from build123d import *

# Parameters (mm, degrees)
BOSS_EXTRUDE2_DEPTH     = 177.8
SKETCH19_R              = 2.2479
CUT_EXTRUDE3_DEPTH      = 27.67
SKETCH21_W              = 3.048
SKETCH21_H              = 14.224
BOSS_EXTRUDE4_DEPTH     = 14.224
SKETCH22_R              = 2.2479
CUT_EXTRUDE4_DEPTH      = 24.622
CUT_EXTRUDE4_DEPTH_BACK = 4.048


with BuildPart() as part:
    # Sketch2 → Boss-Extrude2 (new body)
    with BuildSketch(Plane.XY):
        with BuildLine():
            Line((0, 0), (0, 22.86))
            Line((0, 22.86), (26.67, 22.86))
            Line((26.67, 22.86), (26.67, 0))
            Line((26.67, 0), (23.495, 0))
            Line((23.495, 0), (23.495, 18.542))
            ThreePointArc((23.495, 18.542), (22.974235857, 19.799235857), (21.717, 20.32))
            Line((21.717, 20.32), (4.953, 20.32))
            ThreePointArc((4.953, 20.32), (3.695764143, 19.799235857), (3.175, 18.542))
            Line((3.175, 18.542), (3.175, 0))
            Line((3.175, 0), (0, 0))
        make_face()
    extrude(amount=-BOSS_EXTRUDE2_DEPTH)

    # Sketch19 → Cut-Extrude3 (cut, through all)
    with BuildSketch(Plane(origin=(0, 0, 0), x_dir=(0, 0, -1), z_dir=(1, 0, 0))):
        with Locations((24.13, 9.525)):
            Circle(SKETCH19_R)
        with Locations((64.77, 9.525)):
            Circle(SKETCH19_R)
        with Locations((113.03, 9.525)):
            Circle(SKETCH19_R)
        with Locations((153.67, 9.525)):
            Circle(SKETCH19_R)
    extrude(amount=CUT_EXTRUDE3_DEPTH, mode=Mode.SUBTRACT)

    # Sketch21 → Boss-Extrude4 (add)
    with BuildSketch(Plane(origin=(0, 22.86, 0), x_dir=(1, 0, 0), z_dir=(0, 1, 0))):
        with Locations((1.524, 7.112)):
            Rectangle(SKETCH21_W, SKETCH21_H)
        with Locations((25.146, 7.112)):
            Rectangle(SKETCH21_W, SKETCH21_H)
    extrude(amount=BOSS_EXTRUDE4_DEPTH)

    # Sketch22 → Cut-Extrude4 (cut, two sides)
    with BuildSketch(Plane.ZY.offset(-23.622)) as cut_extrude4_sk:
        with Locations((-7.112, 29.972)):
            Circle(SKETCH22_R)
    extrude(amount=CUT_EXTRUDE4_DEPTH, mode=Mode.SUBTRACT)
    extrude(cut_extrude4_sk.sketch, amount=-CUT_EXTRUDE4_DEPTH_BACK, mode=Mode.SUBTRACT)


solid = part.part
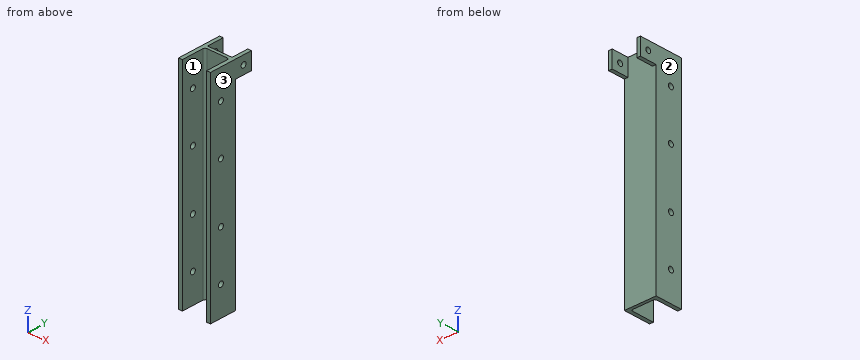
The listing builds one solid part. Answer for the finished solid, in the listing's coordinates (mm). Face numbers are marked on the shaded views. Coordinates: 2 decimals unless noted, no trailing zeros. Write each loop counter-clockwise with the first axis right and the second up, starting at its lowest first coordinate (ties: lowest second). Pieces come first, ordered by that corner, then holes. Notation, with made-up numbers: (14, 78) -> (59, 78) arc R15 cw to (59, 97) -> close; hole circle Ø5 at (-24.75, 60). An arc over 180 degrees is marked (long way). One line per question, with ' | ' between items.
1. For a pull along X with two mould halves and no side action, classify the marked faces 1, 2 and 3 as released by +X, released by -X, zero draft, split by the parting line, or undercut.
Verdict:
face 1: undercut | face 2: released by -X | face 3: released by +X
2. Section B-B (z = -24.13) is taken. Determine the outline of the cut face in (x, y) (3 decimals).
Verdict:
outline: (0, 0) -> (3.175, 0) -> (3.175, 7.277) -> (0, 7.277) -> close; (0, 11.773) -> (3.175, 11.773) -> (3.175, 18.542) arc R1.778 cw to (4.953, 20.32) -> (21.717, 20.32) arc R1.778 cw to (23.495, 18.542) -> (23.495, 11.773) -> (26.67, 11.773) -> (26.67, 22.86) -> (0, 22.86) -> close; (23.495, 0) -> (26.67, 0) -> (26.67, 7.277) -> (23.495, 7.277) -> close
3. Given pin 1 Ø8 at (x, z) = (12.5, -69) entering from +Y; pin 2 Ø13.5 at (x, z) = (15.5, -63.5) entering from -Y, each flat-ended and moving along its own axis, determine where each tip first touches the part or whether it passes through.
Verdict:
pin 1: stops at y = 22.86 | pin 2: stops at y = 20.24
4. Section D-D (y = 34) is taken. Determine the outline of the cut face in (x, z), and give its area (3 significant figures).
Verdict:
outline: (0, -14.22) -> (3.05, -14.22) -> (3.05, 0) -> (0, 0) -> close; (23.62, -14.22) -> (26.67, -14.22) -> (26.67, 0) -> (23.62, 0) -> close | area: 86.7 mm^2
5. Straight lines are drawn through the part: line 1 (X direction, y = 10.5, z = -90) (3 decimals); line 2 (Y direction, x = 1.35, z = -24.13); line 3 (X direction, y = 24.5, z = -7.5). For each, find the intervals that lie inside material, in ascending order.
Verdict:
line 1: x = 0 to 3.175, 23.495 to 26.67 | line 2: y = 0 to 7.28, 11.77 to 22.86 | line 3: x = 0 to 3.05, 23.62 to 26.67
6. Section A-A (y = 14) is taken. Determine the outline of the cut face in (x, z) (3 decimals).
Verdict:
outline: (0, -177.8) -> (3.175, -177.8) -> (3.175, 0) -> (0, 0) -> close; (23.495, -177.8) -> (26.67, -177.8) -> (26.67, 0) -> (23.495, 0) -> close
7. Section C-C (x = 9.25) is taken. Determine the outline of the cut face in (y, z).
Verdict:
outline: (20.32, -177.8) -> (22.86, -177.8) -> (22.86, 0) -> (20.32, 0) -> close
